Autodesk Inventor part; units mm, degrees
ref_plane "YZ Plane" through (0, 0, 0) normal (1, 0, 0) x (0, 1, 0)
ref_plane "XZ Plane" through (0, 0, 0) normal (0, 1, 0) x (-1, 0, 0)
ref_plane "XY Plane" through (0, 0, 0) normal (0, 0, 1) x (1, 0, 0)
sketch "Sketch1" plane through (0, 0, 0) normal (1, 0, 0) x (0, 1, 0)
  circle A0 centre (144, 0) radius 2
  arc A1 (288, 0) -> (288, 0) centre (288, 0) ccw
  circle A2 centre (288, 0) radius 2
  circle A3 centre (0, 0) radius 2
  line L0 (0, 0) -> (288, 0) construction
  line L1 (0, 0) -> (288, 0) construction
  line L2 (0, -12) -> (312, -12)
  line L3 (312, 12) -> (0, 12)
  arc A4 (0, 12) -> (0, -12) centre (0, 0) ccw
  circle A5 centre (9.7, 100) radius 1.6
  circle A6 centre (9.7, 108) radius 4.5
  circle A7 centre (9.7, 116) radius 1.6
  circle A8 centre (9.7, 124) radius 4.5
  circle A9 centre (144, 0) radius 4.5
  circle A10 centre (8, 0) radius 4.35
  circle A11 centre (16, 0) radius 2
  circle A12 centre (24, 0) radius 4.35
  circle A13 centre (32, 0) radius 2
  circle A14 centre (40, 0) radius 4.35
  circle A15 centre (48, 0) radius 2
  circle A16 centre (56, 0) radius 4.35
  circle A17 centre (64, 0) radius 2
  circle A18 centre (72, 0) radius 4.35
  circle A19 centre (80, 0) radius 2
  circle A20 centre (88, 0) radius 4.35
  circle A21 centre (96, 0) radius 2
  circle A22 centre (104, 0) radius 4.35
  circle A23 centre (112, 0) radius 2
  circle A24 centre (120, 0) radius 4.35
  circle A25 centre (128, 0) radius 2
  circle A26 centre (136, 0) radius 4.35
  circle A27 centre (144, 0) radius 2
  circle A28 centre (152, 0) radius 4.35
  circle A29 centre (160, 0) radius 2
  circle A30 centre (168, 0) radius 4.35
  circle A31 centre (176, 0) radius 2
  circle A32 centre (184, 0) radius 4.35
  circle A33 centre (192, 0) radius 2
  circle A34 centre (200, 0) radius 4.35
  circle A35 centre (208, 0) radius 2
  circle A36 centre (216, 0) radius 4.35
  circle A37 centre (224, 0) radius 2
  circle A38 centre (232, 0) radius 4.35
  circle A39 centre (240, 0) radius 2
  circle A40 centre (248, 0) radius 4.35
  circle A41 centre (256, 0) radius 2
  circle A42 centre (264, 0) radius 4.35
  circle A43 centre (272, 0) radius 2
  circle A44 centre (280, 0) radius 4.35
  circle A45 centre (288, 0) radius 2
  circle A46 centre (296, 0) radius 4.35
  circle A47 centre (296, 0) radius 2
  circle A48 centre (304, 0) radius 2
  circle A49 centre (312, 0) radius 2
  arc A50 (312, -12) -> (312, 12) centre (312, 0) ccw
  circle A51 centre (8, 0) radius 2
  circle A52 centre (152, 0) radius 2
  point P0 (148.082969, -1.891921)
  point P1 (139.917031, -1.891921)
  point P2 (139.917031, 1.891921)
  point P3 (148.082969, 1.891921)
  dimension "d0" = 4
  dimension "d1" = 4
  dimension "d2" = 144
  dimension "d3" = 4
  dimension "d4" = 144
  dimension "d6" = 3.2
  dimension "d7" = 9
  dimension "d8" = 8
  dimension "d9" = 8
  dimension "d10" = 8
  dimension "d11" = 9
  dimension "d12" = 8.7
  dimension "d13" = 8
  dimension "d16" = 16
  dimension "d27" = 8
  dimension "d32" = 24
  dimension "d33" = 4
  dimension "d34" = 4
sketch "Sketch1 outline for Extrusion1" plane through (0, 0, 0) normal (1, 0, 0) x (0, 1, 0)
  line L0 (0, -12) -> (312, -12)
  arc A0 (312, -12) -> (312, 12) centre (312, 0) ccw
  line L1 (312, 12) -> (0, 12)
  arc A1 (0, 12) -> (0, -12) centre (0, 0) ccw
  circle A2 centre (0, 0) radius 2
  circle A3 centre (16, 0) radius 2
  circle A4 centre (32, 0) radius 2
  circle A5 centre (48, 0) radius 2
  circle A6 centre (64, 0) radius 2
  circle A7 centre (80, 0) radius 2
  circle A8 centre (96, 0) radius 2
  circle A9 centre (112, 0) radius 2
  circle A10 centre (128, 0) radius 2
  circle A11 centre (160, 0) radius 2
  circle A12 centre (176, 0) radius 2
  circle A13 centre (192, 0) radius 2
  circle A14 centre (208, 0) radius 2
  circle A15 centre (224, 0) radius 2
  circle A16 centre (240, 0) radius 2
  circle A17 centre (256, 0) radius 2
  circle A18 centre (272, 0) radius 2
  circle A19 centre (288, 0) radius 2
  circle A20 centre (296, 0) radius 2
  circle A21 centre (304, 0) radius 2
  circle A22 centre (312, 0) radius 2
  circle A23 centre (8, 0) radius 2
  circle A24 centre (152, 0) radius 2
  circle A25 centre (144, 0) radius 2
extrude "Extrusion1" add sketch "Sketch1 outline for Extrusion1" along normal blind 4.7625
sketch "Sketch1 outline for Extrusion2" plane through (0, 0, 0) normal (1, 0, 0) x (0, 1, 0)
  circle A0 centre (24, 0) radius 4.35
  circle A1 centre (56, 0) radius 4.35
  circle A2 centre (88, 0) radius 4.35
  circle A3 centre (120, 0) radius 4.35
  circle A4 centre (184, 0) radius 4.35
  circle A5 centre (216, 0) radius 4.35
  circle A6 centre (248, 0) radius 4.35
  circle A7 centre (280, 0) radius 4.35
extrude "Extrusion2" add sketch "Sketch1 outline for Extrusion2" against normal blind 1.651 from surface at 0
equation "\"d4\" = d2"
properties part number "Intake Mounting Bracket"
Here's how the part is built. I have some questions about the finished solid (model axes, mm). A direction names the side the tool comes from. Give positions to 0.01 mm unless a question says otherwise; leave off trailing zeros. Loops run counter-clockwise (first coordinate to the right, second up) from the corner with the lowest first, then second, coordinate; pieces in that order, holes last. Notation, with made-up numbers: M 82,63 L 112,63 A25 ccw 112,86 Z; hole C 35,8.25 d5. An arc over 180 degrees is marked long. Put each result on its own line as item: value. Start each with the question number.
(1) If we mould it in two halves opening along Y, with no side actions, what happens to faces 1 (the cylindrical face through (2, 324, 0)), 2 (the flat face through (-1.651, 88, 0)), 3 (the cylindrical face through (-0.814, 188.018, -1.666)), 4 (the cylindrical face through (-0.814, 211.654, 0.191))? For each: +Y half, -Y half, draft (parallel to the pull), parting line (faces both ways), or undercut.
(2) Will these pins go through, and if not, where does the flat tip stop? pin 1 Ø1 at (x, z) = (0, 1) entering from -Y; pin 2 Ø4.5 at (y, z) = (32, 0) entering from -X; pin 3 Ø3 at (y, z) = (0, 0) entering from +X; pin 4 Ø1.5 at (x, z) = (4, -8.5) entering from -Y.
(3) I want a section at A-A on y = 266. Please give me the cut outline in (x, z), then the cut area to 3 significant figures.
(4) I need wall thicknesses on line 1 along Z through (x, y) = (2.95, 240); line 2 along Z through (x, y) = (1, 256.5); line 3 along X through (y, z) = (301, 6.5). Which ranges of each line are inside material? Lowest first, please. Write a range as [from, to].
(5) For faces 5 (the flat face through (-1.651, 184, 0)), 6 (the cylindrical face through (-0.814, 124.018, -1.666)), which set-ups out of +Z, -Z, +X, -X, +Y, -Y let a thin tool reach every point of the face, with its end or its side?
(6) I want a section at B-B on z = 9. Please give me the cut outline in (x, y), then the cut area to 3 significant figures.
Answer block:
1. face 1: +Y half
1. face 2: draft
1. face 3: undercut
1. face 4: undercut
2. pin 1: y = -11.99
2. pin 2: x = 0
2. pin 3: through
2. pin 4: y = -9.16
3. outline: M 0,-12 L 4.76,-12 L 4.76,12 L 0,12 Z
3. area: 114 mm^2
4. line 1: [-12, -2], [2, 12]
4. line 2: [-12, -1.94], [1.94, 12]
4. line 3: [0, 4.76]
5. face 5: +Z, -Z, -X, +Y, -Y
5. face 6: -X
6. outline: M 0,-7.94 L 4.76,-7.94 L 4.76,319.94 L 0,319.94 Z
6. area: 1,560 mm^2
